Model file for the job. Use its own axes, mm. Face numbers are marked on the shaded views. Give positions to 0.01 mm unless a question says otherwise; leave off trailing zeros. Write each loop counter-clockwise with the first axis right and the second up, starting at its lowest first coordinate (ties: lowest second). Pieces come first, ordered by that corner, then holes.
```python
from build123d import *

# Parameters (mm, degrees)
F0_W     = 27.91918
F0_H     = 44.220986
F1_DEPTH = 4.572
F2_R     = 2.908875
F2_R_2   = 3.535422
F2_R_3   = 3.27776
F2_R_4   = 3.027169
F3_DEPTH = 25.4


with BuildPart() as f1:
    # F0 (on Front) → F1 (new body)
    with BuildSketch(Plane.XZ):
        with Locations((-3.466476, -3.560164)):
            Rectangle(F0_W, F0_H)
    extrude(amount=F1_DEPTH)

    # F2 (on Front) → F3 (cut)
    with BuildSketch(Plane.XZ):
        with Locations((-10.305738, 11.430001)):
            Circle(F2_R)
        with Locations((2.248525, -18.362951)):
            Circle(F2_R_2)
        with Locations((-10.493115, -17.426066)):
            Circle(F2_R_3)
        with Locations((2.061148, 11.430001)):
            Circle(F2_R_4)
    extrude(amount=F3_DEPTH, mode=Mode.SUBTRACT)


solid = f1.part
```
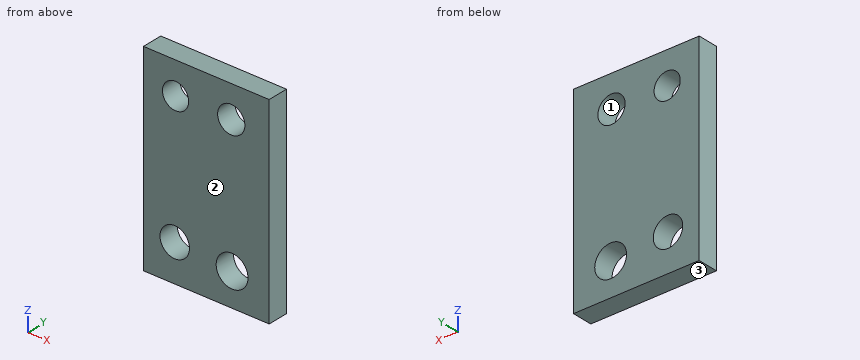
1. Slice it at A-A, the plane z = -19. Write the cut outline in (x, y), and give its area (3 significant figures).
Calculated:
outline: (-17.43, -4.57) - (-13.37, -4.57) - (-13.37, 0) - (-17.43, 0) - close; (-7.62, -4.57) - (-1.23, -4.57) - (-1.23, 0) - (-7.62, 0) - close; (5.73, -4.57) - (10.49, -4.57) - (10.49, 0) - (5.73, 0) - close
area: 69.6 mm2
2. Pull direction Z, two halves, no side cores. Call the marked faces 1, 2 and 3: +Z half, -Z half, draft (parallel to the pull), parting line (faces both ways), or undercut.
Calculated:
face 1: undercut
face 2: draft
face 3: -Z half
3. Slice it at C-C, the plane y = -0.5. Write the cut outline in (x, z), and give its area (3 significant figures).
Calculated:
outline: (-17.43, -25.67) - (10.49, -25.67) - (10.49, 18.55) - (-17.43, 18.55) - close; hole circle Ø6.56 at (-10.49, -17.43); hole circle Ø5.82 at (-10.31, 11.43); hole circle Ø7.07 at (2.25, -18.36); hole circle Ø6.05 at (2.06, 11.43)
area: 1,110 mm2
4. Slice it at B-B, the plane x = -11.75. Write the cut outline in (y, z) (3 decimals), and give its area (3 significant figures).
Calculated:
outline: (-4.572, -25.671) - (0, -25.671) - (0, -20.453) - (-4.572, -20.453) - close; (-4.572, -14.399) - (0, -14.399) - (0, 8.905) - (-4.572, 8.905) - close; (-4.572, 13.955) - (0, 13.955) - (0, 18.55) - (-4.572, 18.55) - close
area: 151 mm2
5. Probe probe 1 along Z at (x, y) = (-8, -2.05); probe 2 along X at (y, z) = (-0.2, 13); probe 3 along X at (y, z) = (-2.5, 10). List the from-to ranges inside material, lowest first.
Calculated:
probe 1: z = -25.67 to -19.55, -15.3 to 9.66, 13.2 to 18.55
probe 2: x = -17.43 to -12.75, -7.86 to -0.53, 4.65 to 10.49
probe 3: x = -17.43 to -12.84, -7.77 to -0.61, 4.73 to 10.49
